Autodesk Inventor part; units mm, degrees
ref_plane "YZ Plane" through (0, 0, 0) normal (1, 0, 0) x (0, 1, 0)
ref_plane "XZ Plane" through (0, 0, 0) normal (0, 1, 0) x (-1, 0, 0)
ref_plane "XY Plane" through (0, 0, 0) normal (0, 0, 1) x (1, 0, 0)
sketch "Boceto10" plane through (0, 0, 0) normal (0, 1, 0) x (-1, 0, 0)
  line L0 (9.2786, 29.6594) -> (9.2786, -404.3406)
  line L1 (9.2786, -404.3406) -> (-105.7214, -404.3406)
  line L2 (-105.7214, -404.3406) -> (-105.7214, 29.6594)
  line L3 (-105.7214, 29.6594) -> (9.2786, 29.6594)
  line L4 (-105.7214, 29.6594) -> (-123.7214, 29.6594)
  line L5 (-123.7214, -404.3406) -> (-105.7214, -404.3406)
  line L6 (9.2786, 29.6594) -> (79.7636, 29.6594)
  line L7 (79.7636, 29.6594) -> (79.7636, -404.3406)
  line L8 (79.7636, -404.3406) -> (9.2786, -404.3406)
  line L9 (-123.7214, 29.6594) -> (-123.7214, -98.0201)
  line L10 (-111.7214, -118.8047) -> (-111.7214, -338.8047)
  line L11 (-123.7214, 29.6594) -> (-123.7214, -98.0201)
  line L12 (-123.7214, -359.5893) -> (-123.7214, -404.3406)
  circle A0 centre (-115.7214, -20.3406) radius 2
  circle A1 centre (-115.7214, -354.3406) radius 2
  line L13 (-111.7214, -118.8047) -> (-123.7214, -98.0201)
  line L14 (-111.7214, -338.8047) -> (-123.7214, -359.5893)
  point P0 (0, 0)
  dimension "d65" = 434
  dimension "d66" = 115
  dimension "d67" = 18
  dimension "d76" = 70.485
  dimension "d77" = 434
  dimension "d108" = 220
  dimension "d125" = 4
  dimension "d126" = 8
  dimension "d127" = 50
  dimension "d128" = 4
  dimension "d129" = 8
  dimension "d130" = 50
  dimension "d133" = 18
  dimension "d166" = 12
extrude "Extrusión13" add sketch "Boceto10" along normal blind 2 contours L0 L1 L2 L3
extrude "Extrusión14" add sketch "Boceto10" along normal blind 2 contours L2 L5 L12 L14 L10 L13 L9 L4
extrude "Extrusión15" add sketch "Boceto10" along normal blind 2 contours L6 L7 L8 L0
bend part "Pieza de plegado2" radius 0.5 angle 90 line through (-9.2786, 0, 29.6594) along (0, 0, -1) centre toward (0, -1, 0) moving side (-1, 0, 0) both sides no
sketch "Boceto11" plane through (-11.7786, -70.1996, -404.3406) normal (-1, 0, 0) x (0, 0, 1)
  line L0 (0, 0) -> (434, 0)
  line L1 (434, 0) -> (434, -194.998)
  line L2 (434, -194.998) -> (0, -194.998)
  line L3 (0, -194.998) -> (0, 0)
  circle A0 centre (17, -30) radius 4
  circle A1 centre (414, -15) radius 5
  point P0 (404.3406, 70.1996)
  dimension "d82" = 194.998
  dimension "d158" = 8
  dimension "d159" = 10
  dimension "d161" = 17
  dimension "d162" = 20
  dimension "d164" = 15
  dimension "d165" = 30
extrude "Extrusión16" add sketch "Boceto11" against normal blind 2
bend part "Pieza de plegado3" radius 0.5 angle 90 line through (-11.7786, -70.1996, -404.3406) along (0, 0, 1) centre toward (-1, 0, 0) moving side (0, -1, 0) both sides no
sketch "Boceto14" plane through (-206.4912, -70.6996, -404.3406) normal (0, 1, 0) x (1, 0, 0)
  line L0 (0, 0) -> (0, -434)
  line L1 (0, -434) -> (-40, -434)
  line L2 (-40, -434) -> (-40, 0)
  line L3 (-40, 0) -> (0, 0)
  line L4 (0, -434) -> (194.2126, -434)
  line L5 (194.2126, 0) -> (0, 0)
  line L6 (0, -434) -> (0, 0)
  point P0 (206.4912, -404.3406)
  dimension "d91" = 40
  dimension "d92" = 434
extrude "Extrusión17" add sketch "Boceto14" against normal blind 2
bend part "Pieza de plegado4" radius 0.5 angle 90 line through (-206.4912, -70.6996, -404.3406) along (0, 0, 1) centre toward (0, 1, 0) moving side (1, 0, 0) both sides no
sketch "Boceto15" plane through (-246.4912, -72.6996, 29.6594) normal (0, -1, 0) x (1, 0, 0)
  line L0 (0, -434) -> (0, 0)
  line L1 (0, -434) -> (8.8, -434)
  line L2 (-29.6996, -434) -> (40, -434)
  circle A0 centre (10, -334) radius 2
  circle A1 centre (10, -100) radius 2
  point P0 (246.4912, -29.6594)
  dimension "d97" = 8.8
  dimension "d98" = 4
  dimension "d99" = 4
  dimension "d101" = 234
  dimension "d102" = 10
  dimension "d103" = 10
  dimension "d136" = 100
extrude "Extrusión18" cut sketch "Boceto15" against normal blind 10
sketch "Boceto16" plane through (-205.9912, -70.1996, 29.6594) normal (-1, 0, 0) x (0, 0, 1)
  circle A0 centre (-135, 111.4272) radius 2
  circle A1 centre (-299, 111.4272) radius 2
  line L0 (0, 193.4272) -> (-434, 193.4272)
  line L1 (0, 0) -> (0, 193.4272)
  line L2 (-434, 193.4272) -> (-434, 0)
  circle A2 centre (-135, 151.4272) radius 2
  circle A3 centre (-299, 151.4272) radius 2
  dimension "d109" = 4
  dimension "d111" = 4
  dimension "d113" = 82
  dimension "d114" = 135
  dimension "d116" = 82
  dimension "d117" = 135
  dimension "d137" = 4
  dimension "d138" = 40
  dimension "d139" = 4
  dimension "d140" = 40
extrude "Extrusión19" cut sketch "Boceto16" against normal blind 10
sketch "Boceto17" plane through (-278.6908, 126.2276, 29.6594) normal (-1, 0, 0) x (0, 0, 1)
  line L0 (0, 0) -> (0, 133)
  line L1 (0, 133) -> (-127.6795, 133)
  circle A0 centre (-319, 114.1) radius 1.5
  circle A1 centre (-310, 114.1) radius 1.5
  line L2 (-434, 133) -> (-434, 0)
  line L3 (-389.2487, 133) -> (-434, 133)
  circle A2 centre (-314.5, 109.5) radius 1.75
  point P0 (-29.6594, -126.2276)
  dimension "d148" = 3
  dimension "d149" = 3
  dimension "d150" = 115
  dimension "d151" = 18.9
  dimension "d152" = 9
  dimension "d153" = 18.9
  dimension "d154" = 3.5
  dimension "d156" = 4.6
  dimension "d157" = 4.5
extrude "Extrusión20" cut sketch "Boceto17" against normal blind 10
equation "\"d67\" = d133"
equation "\"d126\" = d129"
equation "\"d102\" = d103"
equation "\"d116\" = d113"
equation "\"d153\" = d151"
properties part number "Chapon" material "Aluminum 1100-H14"
The model under review builds one solid part; all positions refer to its coordinate system, in mm. A direction names the side the tool comes from. Coordinates: 2 decimals unless noted, no trailing zeros. Write each loop counter-clockwise with the first axis right and the second up, starting at its lowest first coordinate (ties: lowest second). Pieces come first, ordered by that corner, then holes.
1) Machinability: for faces 1 (the face through (-205, 94, 29.659)), 2 (the face through (-227, -70.7, -190)), 3 (the face through (-277.677, 253.144, -349.052)), 4 (the face through (-276.691, 194, -184)), which of the approach directions +Z, -Z, +X, -X, +Y, -Y give a long, thin tool a straight path to every point of the face, cutting with its end or side? Answer none if there is none.
2) To check wall thickness, follow probe 1 along Y at (x, z) = (-209.5, -210); probe 2 along Y at (x, z) = (-253, 1); probe 3 along X at (y, z) = (-6, -57). State the ranges of each line that lie inside material, in increasing order.
3) We need section A-A on z = -323. State the section outline as (x, y) points, then the cut area to 3 significant figures.
4) We need section B-B on x = -228. State the section outline as (y, z) points.
5) We need section D-D on y = 195.5. State the section outline as (x, z) points, then the cut area to 3 significant figures.
6) Clearance check with flat-ended pins moving along their axes: pin 1 Ø21 at (x, z) = (-246.5, -287) entering from +Y; pin 2 Ø1 at (x, z) = (-278, -202.5) entering from +Y; pin 3 Ø3 at (x, z) = (-236.49, -70.34) entering from -Y. State where each tip first meets the part, or that it passes through.
7) The part is to be moulded in two halves that separate along Y. For faces 5 (the face through (-205.5, 94, -404.341)), 6 (the face through (-242, 123.728, -190)), 7 (the face through (-205.991, 25, -190)), 8 (the face through (-277.677, 253.144, -108.558)), say which applies: pulls with the +Y half, pulls with the -Y half, needs draft (parallel to the pull), parting line crosses it, or undercut.
8) We need section C-C on x = -267.5. State the section outline as (y, z) points, then the cut area to 3 significant figures.
Answer list:
1. face 1: +Z, +X, -X, +Y, -Y
1. face 2: +Z, -Z, -X
1. face 3: +X, -X, +Y
1. face 4: +Z, -Z, +X, +Y
2. probe 1: y = -72.7 to -70.7, 123.73 to 125.73
2. probe 2: y = 123.73 to 125.73
2. probe 3: x = -205.99 to -203.99
3. outline: (-278.69, 126.23) arc R2.5 ccw to (-276.19, 123.73) - (-206.49, 123.73) arc R0.5 cw to (-205.99, 123.23) - (-205.99, -70.2) arc R0.5 cw to (-206.49, -70.7) - (-246.49, -70.7) - (-246.49, -72.7) - (-206.49, -72.7) arc R2.5 ccw to (-203.99, -70.2) - (-203.99, 123.23) arc R2.5 ccw to (-206.49, 125.73) - (-276.19, 125.73) arc R0.5 cw to (-276.69, 126.23) - (-276.69, 247.23) - (-278.69, 247.23) - close
3. area: 862 mm2
4. outline: (-72.7, -404.34) - (-70.7, -404.34) - (-70.7, 29.66) - (-72.7, 29.66) - close; (123.73, -404.34) - (125.73, -404.34) - (125.73, 29.66) - (123.73, 29.66) - close
5. outline: (-278.69, -404.34) - (-276.69, -404.34) - (-276.69, 29.66) - (-278.69, 29.66) - close
5. area: 868 mm2
6. pin 1: stops at y = 125.73
6. pin 2: stops at y = 247.23
6. pin 3: stops at y = 123.73
7. face 5: needs draft
7. face 6: undercut
7. face 7: undercut
7. face 8: pulls with the +Y half
8. outline: (123.73, -404.34) - (125.73, -404.34) - (125.73, 29.66) - (123.73, 29.66) - close
8. area: 868 mm2
